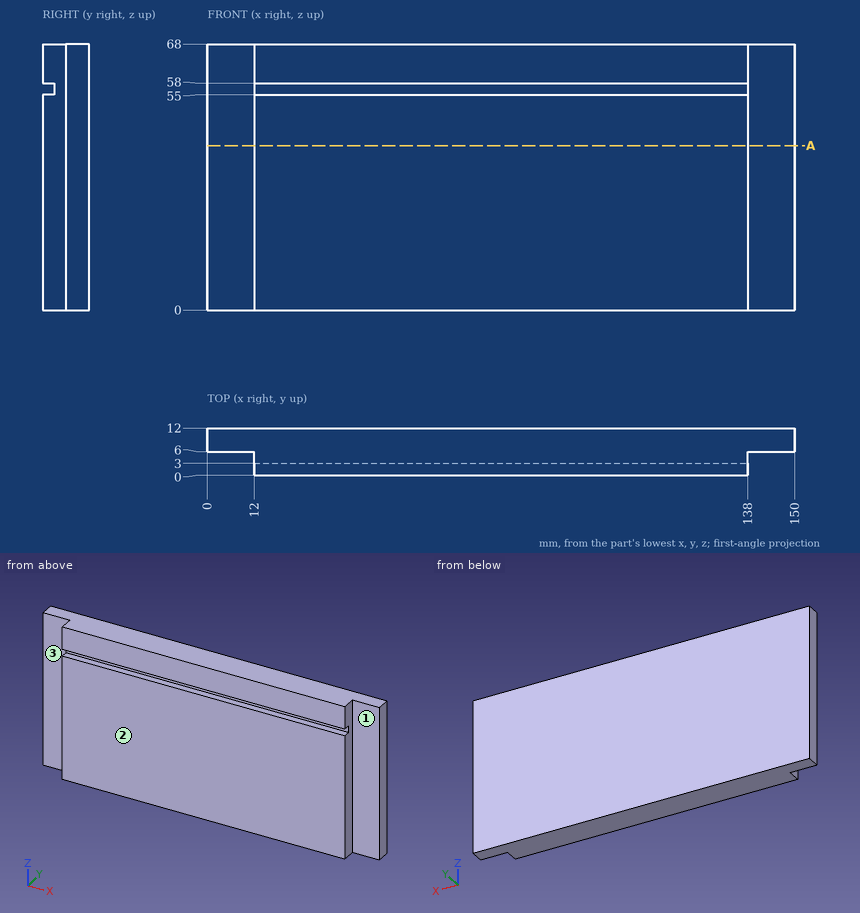
Print and shaded views of the part. All mm, measured from the part's lowest x, y and z. A direction names the side the tool comes from. Give positions to 0.01 mm unless a question says otherwise; leave off trailing zeros. Loops run counter-clockwise (first coordinate to the right, second up) from the corner with the lowest first, then second, coordinate; pieces in that order, holes last. Notation, with made-up numbers: M -39.75,16.5 L -28.75,16.5 A27 cw -28.75,49.5 Z; hole C 23.5,22 d10. An arc over 180 degrees is marked long. Write each question's results on one line, items separated by ' | '.
Q1. Probe probe 1 along Z at (x, y) = (113, 2.75); probe 2 along X at (y, z) = (5, 50); probe 3 along Y at (x, z) = (94, 56.5). List the from-to ranges inside material, lowest first.
Geometry check:
probe 1: z = 0 to 55, 58 to 68 | probe 2: x = 12 to 138 | probe 3: y = 3 to 12
Q2. Which spindle directions (+Z, -Z, +X, -X, +Y, -Y) get a long thin tool onto all of the face, cutting with end or side? Do the marked faces 1, 2 and 3. Say none if no direction does.
Geometry check:
face 1: +Z, -Z, +X, -Y | face 2: +Z, -Z, +X, -X, -Y | face 3: +Z, -Z, -X, -Y
Q3. Flat gauge pins, fed straight in: P1, Ø3.5, axis at x = 144, z = 35.5, coming from the -Y side; P2, Ø6, axis at y = 1.5, z = 51, coming from the +X side. Where does each tip first touch, or does it go through?
Geometry check:
P1: stops at y = 6 | P2: stops at x = 138
Q4. Band-saw the part on A-A on z = 42. Write the cut outline in (x, y).
Geometry check:
outline: M 0,6 L 12,6 L 12,0 L 138,0 L 138,6 L 150,6 L 150,12 L 0,12 Z
